Could you check a few things on this model? Use its own coordinates, in mm. A direction names the side the tool comes from. Round coordinates to 2 decimals unless told otherwise and drop trailing zeros. Loops run counter-clockwise (first coordinate to the right, second up) from the corner with the lowest first, then second, coordinate; pieces in that order, holes last. Notation, with made-up numbers: (-25.75, 77) -> (25.25, 77) arc R25 ccw to (25.25, 113) -> close; hole circle Ø5 at (68.5, 4.5). An arc over 180 degrees is marked (long way). Write each question's results on one line, items separated by ' | '.
from build123d import *

# Parameters (mm, degrees)
F0_R     = 19.05
F1_DEPTH = 69.85
F2_R     = 12.7
F3_DEPTH = 63.5
F5_DEPTH = 6.35
F6_R     = 4.7625
F7_DEPTH = 69.851


with BuildPart() as f1:
    # F0 (on Top) → F1 (new body)
    with BuildSketch(Plane.XY):
        Circle(F0_R)
    extrude(amount=F1_DEPTH)

    # F2 (on face) → F3 (cut)
    with BuildSketch(Plane.XY.offset(69.85)):
        Circle(F2_R)
    extrude(amount=-F3_DEPTH, mode=Mode.SUBTRACT)

    # F4 (on face) → F5 (join)
    with BuildSketch(Plane.XY.offset(69.85)):
        with BuildLine():
            Line((50.8, 19.05), (3.68e-08, 19.05))
            ThreePointArc((3.68e-08, 19.05), (13.4703841946, 13.4703841686), (19.05, 0))
            ThreePointArc((19.05, 0), (13.4703841946, -13.4703841686), (3.68e-08, -19.05))
            Line((3.68e-08, -19.05), (50.8, -19.05))
            Line((50.8, -19.05), (50.8, -9.652))
            Line((50.8, -9.652), (35.052, -9.652))
            ThreePointArc((35.052, -9.652), (25.4, 0), (35.052, 9.652))
            Line((35.052, 9.652), (50.8, 9.652))
            Line((50.8, 9.652), (50.8, 19.05))
        make_face()
        with BuildLine():
            Line((3.68e-08, 19.05), (-50.8, 19.05))
            Line((-50.8, 19.05), (-50.8, 9.652))
            Line((-50.8, 9.652), (-35.052, 9.652))
            ThreePointArc((-35.052, 9.652), (-25.4, 0), (-35.052, -9.652))
            Line((-35.052, -9.652), (-50.8, -9.652))
            Line((-50.8, -9.652), (-50.8, -19.05))
            Line((-50.8, -19.05), (3.68e-08, -19.05))
            ThreePointArc((3.68e-08, -19.05), (-19.05, 0), (3.68e-08, 19.05))
        make_face()
    extrude(amount=-F5_DEPTH)

    # F6 (on face) → F7 (cut, through all)
    with BuildSketch(Plane(origin=(0, 0, 0), x_dir=(1, 0, 0), z_dir=(0, 0, -1))):
        Circle(F6_R)
    extrude(amount=-F7_DEPTH, mode=Mode.SUBTRACT)


solid = f1.part
1) I'm going to push flat-ended pins straight in: pin 1 (8 mm diameter, centred on y = 5.5, z = 44.5, fed in from -X); pin 2 (1.5 mm diameter, centred on y = -11.5, z = 54.5, fed in from -X); pin 3 (12 mm diameter, centred on y = 9.5, z = 30.5, fed in from -X). Where does each tip first touch, or does it pass through?
Model answer:
pin 1: stops at x = -18.99 | pin 2: stops at x = -15.73 | pin 3: stops at x = -18.73
2) I want a section at B-B, the plane x = 37.5. Write out the boundary of the cut face in (y, z).
Model answer:
outline: (-19.05, 63.5) -> (-9.65, 63.5) -> (-9.65, 69.85) -> (-19.05, 69.85) -> close; (9.65, 63.5) -> (19.05, 63.5) -> (19.05, 69.85) -> (9.65, 69.85) -> close
3) I want a section at A-A, the plane y = 0. Write out the boundary of the cut face in (x, z).
Model answer:
outline: (-25.4, 63.5) -> (-19.05, 63.5) -> (-19.05, 0) -> (-4.76, 0) -> (-4.76, 6.35) -> (-12.7, 6.35) -> (-12.7, 69.85) -> (-25.4, 69.85) -> close; (4.76, 0) -> (19.05, 0) -> (19.05, 63.5) -> (25.4, 63.5) -> (25.4, 69.85) -> (12.7, 69.85) -> (12.7, 6.35) -> (4.76, 6.35) -> close
4) I need wall thicknesses on line 1 (Y direction, x = 0, z = 3.5); line 2 (X direction, y = 0.5, z = 32). Which ranges of each line are inside material? Lowest first, please.
Model answer:
line 1: y = -19.05 to -4.76, 4.76 to 19.05 | line 2: x = -19.04 to -12.69, 12.69 to 19.04
5) I want a section at D-D, the plane x = 6.5. Write out the boundary of the cut face in (y, z), plus the area to 3 significant figures.
Model answer:
outline: (-19.05, 63.5) -> (-17.91, 63.5) -> (-17.91, 0) -> (17.91, 0) -> (17.91, 63.5) -> (19.05, 63.5) -> (19.05, 69.85) -> (10.91, 69.85) -> (10.91, 6.35) -> (-10.91, 6.35) -> (-10.91, 69.85) -> (-19.05, 69.85) -> close | area: 1,130 mm2
6) For faces 5 (the flat face through (-1, -19.05, 67)), 6 (the cylindrical face through (-2.75, -12.4, 38.54)), 7 (the flat face through (43, -9.652, 67)), 8 (the flat face through (-50.8, 14, 67)), 9 (the flat face through (-43, 9.652, 67)), which set-ups out of +Z, -Z, +X, -X, +Y, -Y let a thin tool reach every point of the face, with its end or its side?
Model answer:
face 5: +Z, -Z, +X, -X, -Y | face 6: +Z | face 7: +Z, -Z, +X | face 8: +Z, -Z, -X, +Y, -Y | face 9: +Z, -Z, -X
7) I want a section at C-C, the plane z = 14.5. Write out the boundary of the cut face in (x, y), plus the area to 3 significant figures.
Model answer:
outline: circle Ø38.1 at (0, 0); hole circle Ø25.4 at (0, 0) | area: 633 mm2
8) If we mould it in two halves opening along Y, with no side actions, what happens to faces 1 (the flat face through (50.8, 14, 67)), 2 (the flat face through (-43, -9.652, 67)), 3 (the flat face through (1, 19.05, 67)), 4 (the cylindrical face through (-15.12, -11.59, 31.31))? For each: released by +Y, released by -Y, zero draft, split by the parting line, or undercut.
Model answer:
face 1: zero draft | face 2: undercut | face 3: released by +Y | face 4: split by the parting line
